from build123d import *

# Parameters (mm, degrees)
BOSS_EXTRUDE1_DEPTH = 7
SKETCH2_W           = 44.9
SKETCH2_H           = 67
CUT_EXTRUDE1_DEPTH  = 10
SKETCH3_R           = 1.9
CUT_EXTRUDE2_DEPTH  = 15
CHAMFER1_SIZE       = 1
SKETCH2_3_W         = 2
SKETCH2_3_H         = 15
CUT_EXTRUDE5_DEPTH  = 4
SKETCH7_W           = 2
SKETCH7_H           = 15
BOSS_EXTRUDE2_DEPTH = 1
CUT_EXTRUDE7_DEPTH  = 15
SKETCH11_W          = 7.1
SKETCH11_H          = 26
CUT_EXTRUDE9_DEPTH  = 6
CUT_EXTRUDE10_DEPTH = 10
SKETCH15_W          = 7.1
SKETCH15_H          = 1.45
BOSS_EXTRUDE3_DEPTH = 1


with BuildPart() as part:
    # Sketch1 → Boss-Extrude1 (new body, symmetric)
    with BuildSketch(Plane(origin=(0, 0, 0), x_dir=(1, 0, 0), z_dir=(0, 1, 0))):
        with BuildLine():
            ThreePointArc((-36.5, -32.5), (-36.358942749, -33.552882169), (-35.945719569, -34.531506006))
            Line((-35.945719569, -34.531506006), (0, 1.414213562))
            Line((0, 1.414213562), (-34.531506006, 35.945719569))
            ThreePointArc((-34.531506006, 35.945719569), (-35.973184708, 34.484184464), (-36.5, 32.5))
            Line((-36.5, 32.5), (-36.5, -32.5))
        make_face()
        with BuildLine():
            Line((-34.531506006, 35.945719569), (0, 1.414213562))
            Line((0, 1.414213562), (34.531506006, 35.945719569))
            ThreePointArc((34.531506006, 35.945719569), (33.552882169, 36.358942749), (32.5, 36.5))
            Line((32.5, 36.5), (-32.5, 36.5))
            ThreePointArc((-32.5, 36.5), (-33.552882169, 36.358942749), (-34.531506006, 35.945719569))
        make_face()
        with BuildLine():
            Line((0, 1.414213562), (35.945719569, -34.531506006))
            ThreePointArc((35.945719569, -34.531506006), (36.358942749, -33.552882169), (36.5, -32.5))
            Line((36.5, -32.5), (36.5, 32.5))
            ThreePointArc((36.5, 32.5), (35.973184708, 34.484184464), (34.531506006, 35.945719569))
            Line((34.531506006, 35.945719569), (0, 1.414213562))
        make_face()
        with BuildLine():
            ThreePointArc((-35.945719569, -34.531506006), (-34.484184464, -35.973184708), (-32.5, -36.5))
            Line((-32.5, -36.5), (32.5, -36.5))
            ThreePointArc((32.5, -36.5), (34.484184464, -35.973184708), (35.945719569, -34.531506006))
            Line((35.945719569, -34.531506006), (0, 1.414213562))
            Line((0, 1.414213562), (-35.945719569, -34.531506006))
        make_face()
    extrude(amount=BOSS_EXTRUDE1_DEPTH, both=True)

    # Sketch2 → Cut-Extrude1 (cut)
    with BuildSketch(Plane.XZ.offset(7)):
        with Locations((-3.95, 0)):
            Rectangle(SKETCH2_W, SKETCH2_H)
        with BuildLine():
            Line((18.5, 33.5), (18.5, -33.5))
            Line((18.5, -33.5), (18.5, -36.5))
            Line((18.5, -36.5), (32.5, -36.5))
            ThreePointArc((32.5, -36.5), (35.328427125, -35.328427125), (36.5, -32.5))
            Line((36.5, -32.5), (36.5, 32.5))
            ThreePointArc((36.5, 32.5), (35.328427125, 35.328427125), (32.5, 36.5))
            Line((32.5, 36.5), (18.5, 36.5))
            Line((18.5, 36.5), (18.5, 33.5))
        make_face()
    extrude(amount=-CUT_EXTRUDE1_DEPTH, mode=Mode.SUBTRACT)

    # Sketch3 → Cut-Extrude2 (cut, through all)
    with BuildSketch(Plane.XZ.offset(7)):
        with Locations((-29.9, 3)):
            Circle(SKETCH3_R)
        with Locations((-29.9, -3)):
            Circle(SKETCH3_R)
    extrude(amount=-CUT_EXTRUDE2_DEPTH, mode=Mode.SUBTRACT)

    # Chamfer1
    chamfer1_edges = [part.edges().sort_by_distance(p)[0] for p in [
        (-31.8, 7, 3),
        (-31.8, 7, -3),
    ]]
    chamfer(chamfer1_edges, length=CHAMFER1_SIZE)

    # Sketch2<3> → Cut-Extrude5 (cut)
    with BuildSketch(Plane.XZ.offset(7)):
        Polygon((-33.5, -7.5), (-33.5, -33.5), (-26.4, -33.5), (-26.4, 33.5), (-33.5, 33.5), (-33.5, 7.5), align=None)
        with Locations((-34.5, 0)):
            Rectangle(SKETCH2_3_W, SKETCH2_3_H)
    extrude(amount=-CUT_EXTRUDE5_DEPTH, mode=Mode.SUBTRACT)

    # Sketch7 → Boss-Extrude2 (add)
    with BuildSketch(Plane.XZ.offset(3)):
        with Locations((-34.5, 0)):
            Rectangle(SKETCH7_W, SKETCH7_H)
    extrude(amount=BOSS_EXTRUDE2_DEPTH)

    # Sketch9 → Cut-Extrude7 (cut, through all)
    with BuildSketch(Plane(origin=(0, 7, 0), x_dir=(1, 0, 0), z_dir=(0, 1, 0))):
        with BuildLine():
            Line((32.5, 36.5), (22.5, 36.5))
            ThreePointArc((22.5, 36.5), (27.5, 31.5), (32.5, 36.5))
        make_face()
    extrude(amount=-CUT_EXTRUDE7_DEPTH, mode=Mode.SUBTRACT)

    # Sketch11 → Cut-Extrude9 (cut)
    with BuildSketch(Plane.XZ.offset(3)):
        with Locations((-29.95, 20.5)):
            Rectangle(SKETCH11_W, SKETCH11_H)
        with Locations((-29.95, -20.5)):
            Rectangle(SKETCH11_W, SKETCH11_H)
    extrude(amount=-CUT_EXTRUDE9_DEPTH, mode=Mode.SUBTRACT)

    # Sketch13 → Cut-Extrude10 (cut)
    with BuildSketch(Plane.XZ.offset(7)):
        with BuildLine():
            Line((-32.5, -36.5), (18.5, -36.5))
            Line((18.5, -36.5), (18.5, -33.5))
            Line((18.5, -33.5), (-33.5, -33.5))
            Line((-33.5, -33.5), (-33.5, -7.5))
            Line((-33.5, -7.5), (-35.5, -7.5))
            Line((-35.5, -7.5), (-35.5, 7.5))
            Line((-35.5, 7.5), (-33.5, 7.5))
            Line((-33.5, 7.5), (-33.5, 33.5))
            Line((-33.5, 33.5), (18.5, 33.5))
            Line((18.5, 33.5), (18.5, 36.5))
            Line((18.5, 36.5), (-32.5, 36.5))
            ThreePointArc((-32.5, 36.5), (-35.328427125, 35.328427125), (-36.5, 32.5))
            Line((-36.5, 32.5), (-36.5, -32.5))
            ThreePointArc((-36.5, -32.5), (-35.328427125, -35.328427125), (-32.5, -36.5))
        make_face()
    extrude(amount=-CUT_EXTRUDE10_DEPTH, mode=Mode.SUBTRACT)

    # Sketch15 → Boss-Extrude3 (add)
    with BuildSketch(Plane.XZ.offset(3)):
        with Locations((-29.95, -6.775)):
            Rectangle(SKETCH15_W, SKETCH15_H)
    extrude(amount=BOSS_EXTRUDE3_DEPTH)


solid = part.part
Design review of the part built by this model. Coordinates are the model's own, in mm. A direction names the side the tool comes from. Round coordinates to 2 decimals unless told otherwise and drop trailing zeros. Loops run counter-clockwise (first coordinate to the right, second up) from the corner with the lowest first, then second, coordinate; pieces in that order, holes last. Notation, with made-up numbers: M 85.25,-29 L 99.25,-29 A12 ccw 99.25,-14 Z; hole C 83,29.5 d1. An arc over 180 degrees is marked long. Answer as a JSON object with one key per item and string values.
Item 1: We need section B-B on x = -29.9. Give the boundary of the cut face in (y, z), and give its area (3 significant figures).
Answer sheet:
{"outline": "M -4,-7.5 L 3,-7.5 L 3,-36.5 L 7,-36.5 L 7,-5.9 L 6,-4.9 L -3,-4.9 L -3,-6.05 L -4,-6.05 Z; M -3,-1.1 L 6,-1.1 L 7,-0.1 L 7,0.1 L 6,1.1 L -3,1.1 Z; M -3,4.9 L 6,4.9 L 7,5.9 L 7,36.5 L 3,36.5 L 3,7.5 L -3,7.5 Z", "area": "305 mm^2"}
Item 2: We need section D-D on x = -10.5. Give the boundary of the cut face in (y, z).
Answer sheet:
{"outline": "M 3,-36.5 L 7,-36.5 L 7,36.5 L 3,36.5 Z"}
Item 3: Wall thickness on L1, parallel to Z at x = -29.9, y = 1; L2, parallel to Y at x = 17.5, z = 29; L3, parallel to Z at x = -27, y = -1: over which ranges is each line inside the solid? List them lowest first. Write a range as from..to.
Answer sheet:
{"L1": "z = -7.5..-4.9, -1.1..1.1, 4.9..7.5", "L2": "y = 3..7", "L3": "z = -7.5..7.5"}
Item 4: We need section C-C on y = -1.25. Give the boundary of the cut face in (x, z), and give its area (3 significant figures).
Answer sheet:
{"outline": "M -35.5,-7.5 L -26.4,-7.5 L -26.4,7.5 L -35.5,7.5 Z; hole C -29.9,-3 d3.8; hole C -29.9,3 d3.8", "area": "114 mm^2"}
Item 5: Machinability: for faces 4 (the flat face through (-35.5, -1, 0)), 5 (the flat face through (-30, -3, 0.8)), 6 (the flat face through (-26.4, 0, 0)), which of the approach directions +Z, -Z, +X, -X, +Y, -Y give a long, thin tool a straight path to every point of the face, cutting with its end or side? Answer none if there is none.
Answer sheet:
{"face 4": "+Z, -Z, -X, -Y", "face 5": "+Z, +X, -Y", "face 6": "+Z, -Z, +X, -Y"}
Item 6: Clearance check with flat-ended pins moving along their axes: P1, Ø1.5, axis at x = -16, z = -19.5, coming from the -Y side; P2, Ø2.5, axis at x = -29.9, z = 3, coming from the -Y side; P3, Ø3.5, axis at y = -0.5, z = 0, coming from the +X side; P4, Ø0.8, axis at y = -3.5, z = -1.5, coming from the +X side. State where each tip first meets the part, or that it passes through.
Answer sheet:
{"P1": "stops at y = 3", "P2": "passes through", "P3": "stops at x = -26.4", "P4": "stops at x = -33.5"}
Item 7: We need section A-A on z = 3. Give the boundary of the cut face in (x, y), and give its area (3 significant figures).
Answer sheet:
{"outline": "M -36.5,3 L -35.5,3 L -35.5,-4 L -33.5,-4 L -33.5,-3 L -31.8,-3 L -31.8,6 L -32.8,7 L -36.5,7 Z; M -28,-3 L -26.4,-3 L -26.4,3 L 36.5,3 L 36.5,7 L -27,7 L -28,6 Z", "area": "310 mm^2"}
Item 8: The part is to be moulded in two halves that separate along Z. For faces 1 (the flat face through (-1, 7, -1)), 2 (the cylindrical face through (-31.8, 1.44, -2.92)), 3 (the flat face through (-31, -1, 7.5)), say which applies: pulls with the +Z half, pulls with the -Z half, needs draft (parallel to the pull), parting line crosses it, or undercut.
Answer sheet:
{"face 1": "needs draft", "face 2": "undercut", "face 3": "pulls with the +Z half"}
